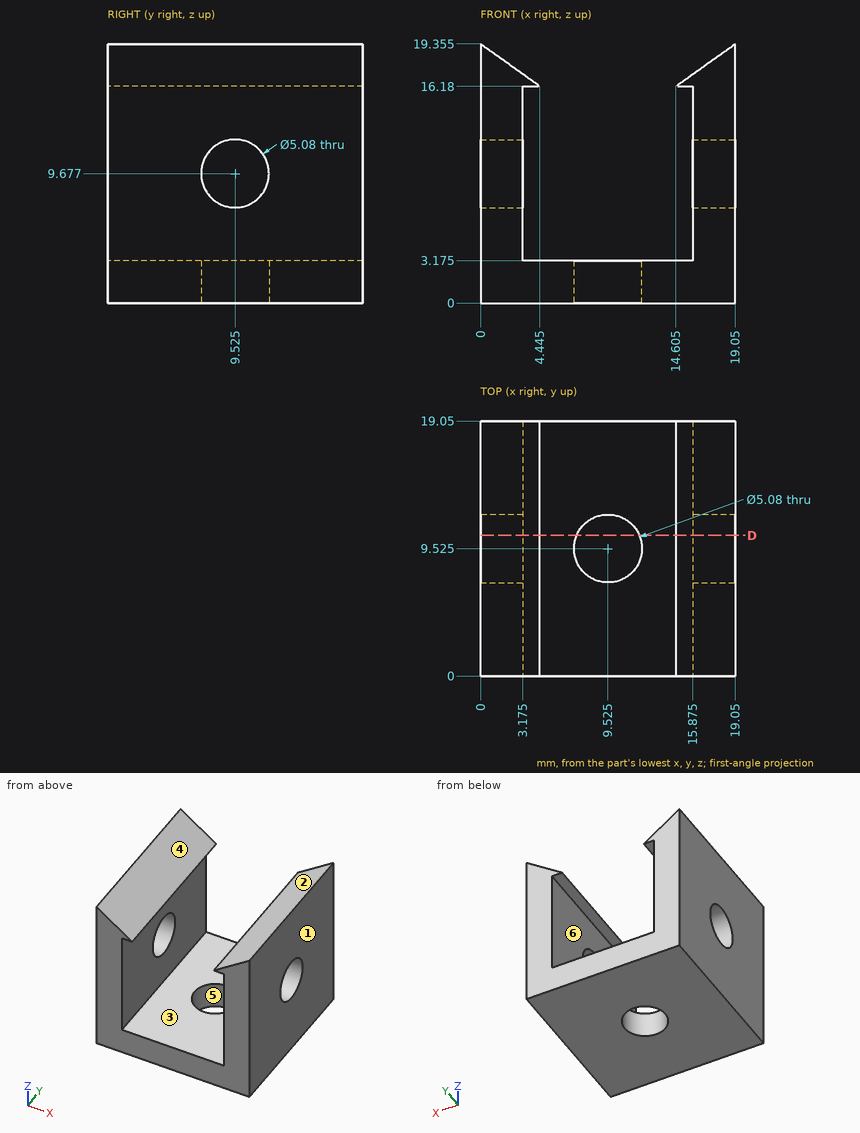
Here's the drawing with two shaded views (mm, measured from the low corner). I have some questions. A direction names the side the tool comes from. Give positions to 0.01 mm unless a question says otherwise; leave off trailing zeros. Use a Markdown table: item, result. Add a question column.
Item 1: For the marked faces 1, 2 and 3, which set-ups out of +Z, -Z, +X, -X, +Y, -Y let a thin tool reach every point of the face, with its end or its side?
Item 2: Imagine slicing it at D-D on y = 10.5. Give the number of separate pieces and of enclosed holes in the cut face.
Item 3: If we mould it in two halves opening along Z, with no side actions, what happens to the marked faces 4, 5 and 6? For each: pulls with the +Z half, pulls with the -Z half, needs draft (parallel to the pull), parting line crosses it, or undercut.
Item 4: I need wall thicknesses on line 1 (Z direction, x = 7.25, y = 1.25) (1 decimal); line 2 (Z direction, x = 2, y = 4) (1 decimal); line 3 (Z direction, x = 3.75, y = 5.75) (1 decimal). Which ranges of each line are inside material? Lowest first, please.
Item 5: Will these pins go through, and if not, where does the flat tip stop? pin 1 (8 mm diameter, centred on x = 15.5, z = 16, fed in from -Y); pin 2 (4.5 mm diameter, centred on x = 9.525, y = 9.525, fed in from -Z).
Data:
| question | item | result |
|---|---|---|
| 1 | face 1 | +Z, -Z, +X, +Y, -Y |
| 1 | face 2 | +Z, +Y, -Y |
| 1 | face 3 | +Y, -Y |
| 2 | separate pieces | 4 |
| 2 | enclosed holes | 0 |
| 3 | face 4 | pulls with the +Z half |
| 3 | face 5 | needs draft |
| 3 | face 6 | undercut |
| 4 | line 1 | z = 0 to 3.2 |
| 4 | line 2 | z = 0 to 17.9 |
| 4 | line 3 | z = 0 to 3.2, 16.2 to 16.7 |
| 5 | pin 1 | stops at y = 0 |
| 5 | pin 2 | passes through |
